Input: part model. Units: mm. Frame: model coordinates. A direction names the side the tool comes from. Coordinates: 2 decimals unless noted, no trailing zeros. Write each loop counter-clockwise with the first axis right and the second up, starting at its lowest first coordinate (ties: lowest second). Pieces come first, ordered by that corner, then holes. Notation, with made-up numbers: (-4, 22) - (46, 22) arc R8 cw to (46, 31) - close; hole circle Ø5 at (-3.5, -24.5). An arc over 180 degrees is marked (long way). Use a Markdown table: item, result. Add a question column.
Q1. Material intervals for probe 1 along Y at (x, z) = (3.5, 0.65); probe 2 along Z at (x, y) = (4.75, 0.6); probe 3 along X at (y, z) = (4.25, 2), sorted ascending. Write a range as from..to.
Q2. Pin query (flat end, axial travel): P1, Ø2, axis at x = 6, z = 1.5, coming from the -Y side; P2, Ø3, axis at x = 2, y = 2, coming from the +Z side. Return the tip coordinate at first contact, or that it passes through.
Q3. Section query A-A (z = 4.5). Return the cut outline in (x, y).
Q4. Section query B-B (x = 3.5). Return the cut outline in (y, z).
Q5. Section query D-D (y = 0.4). Return the cut outline in (x, z), then the cut area to 3 significant figures.
Q6. Mould query, pull axis Z, two halves, no side actions, for faces 1 (the face through (6.699, 2.535, 0.285)), 2 (the face through (6.86, 2.46, 7.51)), 3 (the face through (6.3, 5, 2.7)), 4 (the face through (6.49, 1.07, 4.95)). Classes: released by +Z, released by -Z, zero draft, split by the parting line, or undercut.
Q7. Set-up query: faces 5 (the face through (5, 4, 0)), 6 (the face through (1.6, 2.5, 1)). Return all of +Z, -Z, +X, -X, +Y, -Y with unobstructed straight access to the full face (end or side cutting, diameter ignored); none if empty.
Q8. Section query C-C (y = 3.8). Return the cut outline in (x, z).
from build123d import *

# Parameters (mm, degrees)
SKETCH1_W           = 7
SKETCH1_H           = 5
SKETCH1_R           = 1.5
BOSS_EXTRUDE1_DEPTH = 1
SKETCH2_W           = 1
SKETCH2_H           = 5
BOSS_EXTRUDE2_DEPTH = 7
SKETCH3_R           = 1.5
CUT_EXTRUDE1_DEPTH  = 1
FILLET1_R           = 1
FILLET4_R           = 1
FILLET5_R           = 1


# Some blends are built 0.0001 mm under size
with BuildPart() as part:
    # Sketch1 → Boss-Extrude1 (new body)
    with BuildSketch(Plane.XY):
        with Locations((3.5, 2.5)):
            Rectangle(SKETCH1_W, SKETCH1_H)
        with Locations((3.5, 2.5)):
            Circle(SKETCH1_R, mode=Mode.SUBTRACT)
    extrude(amount=BOSS_EXTRUDE1_DEPTH)

    # Sketch2 → Boss-Extrude2 (add)
    with BuildSketch(Plane.XY.offset(1)):
        with Locations((6.5, 2.5)):
            Rectangle(SKETCH2_W, SKETCH2_H)
    extrude(amount=BOSS_EXTRUDE2_DEPTH)

    # Sketch3 → Cut-Extrude1 (cut)
    with BuildSketch(Plane.ZY.offset(-6)):
        with Locations(Location((4.5, 2.5, 0), (0, 0, 270))):
            Circle(SKETCH3_R)
    extrude(amount=-CUT_EXTRUDE1_DEPTH, mode=Mode.SUBTRACT)

    # Fillet1
    fillet1_edges = [part.edges().sort_by_distance(p)[0] for p in [
        (6, 2.5, 1),
    ]]
    fillet(fillet1_edges, radius=FILLET1_R - 0.0001)  # a hair under: the kernel refuses the full size

    # Fillet4
    # the kernel refuses this fillet: 1 mm, written as the material it takes off along each edge
    with BuildSketch(Plane(origin=(7, -2.5, 8), x_dir=(-1, 0, 0), z_dir=(0, 1, 0)), Plane(origin=(0, 7.5, 1), x_dir=(1, 0, 0), z_dir=(0, -1, 0)), Plane(origin=(0, 7.5, 0), x_dir=(0, 0, 1), z_dir=(0, -1, 0))) as fillet4_piece_1:
        with BuildLine():
            CenterArc((FILLET4_R, -FILLET4_R), FILLET4_R, 90, 90)
            Line((0, -FILLET4_R), (0, 0))
            Line((0, 0), (FILLET4_R, 0))
        make_face()
    extrude(amount=10, mode=Mode.SUBTRACT)
    with BuildSketch(Plane(origin=(6, 7.5, 8), x_dir=(0, 0, -1), z_dir=(0, -1, 0))) as fillet4_piece_2:
        with BuildLine():
            CenterArc((FILLET4_R, FILLET4_R), FILLET4_R, 180, 90)
            Line((0, FILLET4_R), (0, 0))
            Line((0, 0), (FILLET4_R, 0))
        make_face()
    extrude(amount=10, mode=Mode.SUBTRACT)

    # Fillet5
    fillet5_edges = [part.edges().sort_by_distance(p)[0] for p in [
        (7, 2.5, 0),
    ]]
    fillet(fillet5_edges, radius=FILLET5_R)


solid = part.part
Values follow:
| question | item | result |
|---|---|---|
| 1 | probe 1 | 0..1, 4..5 |
| 1 | probe 2 | 0..1 |
| 1 | probe 3 | 6..7 |
| 2 | P1 | y = 0 |
| 2 | P2 | z = 1 |
| 3 | outline | (6, 0) - (7, 0) - (7, 1) - (6, 1) - close; (6, 4) - (7, 4) - (7, 5) - (6, 5) - close |
| 4 | outline | (0, 0) - (1, 0) - (1, 1) - (0, 1) - close; (4, 0) - (5, 0) - (5, 1) - (4, 1) - close |
| 5 | outline | (0.13, 0.5) arc R1 ccw to (1, 0) - (6, 0) arc R1 ccw to (7, 1) - (7, 7) arc R1 ccw to (6.5, 7.87) arc R1 ccw to (6, 7) - (6, 2) arc R1 cw to (5, 1) - (1, 1) arc R1 ccw to start |
| 5 | area | 13.2 mm2 |
| 6 | face 1 | released by -Z |
| 6 | face 2 | released by +Z |
| 6 | face 3 | zero draft |
| 6 | face 4 | undercut |
| 7 | face 5 | -Z, +X, -X, +Y, -Y |
| 7 | face 6 | +Z, -X, +Y, -Y |
| 8 | outline | (0.13, 0.5) arc R1 ccw to (1, 0) - (2.75, 0) - (2.75, 1) - (1, 1) arc R1 ccw to start; (4.25, 0) - (6, 0) arc R1 ccw to (7, 1) - (7, 3.75) - (6, 3.75) - (6, 2) arc R1 cw to (5, 1) - (4.25, 1) - close; (6, 5.25) - (7, 5.25) - (7, 7) arc R1 ccw to (6.5, 7.87) arc R1 ccw to (6, 7) - close |
